The figure shows three views and two pictorial views of one solid part (mm, origin at its lowest corner). Answer the questions. Give positions to 0.01 mm unless a question says otherwise; leave off trailing zeros. Loops run counter-clockwise (first coordinate to the right, second up) from the corner with the lowest first, then second, coordinate; pieces in that order, holes last. Notation, with made-up numbers: (34.5, 54.25) - (41.5, 54.25) arc R21 ccw to (41.5, 78.25) - close; hole circle Ø11 at (-3.75, 59). An arc over 180 degrees is marked (long way). Use CSV: the item, a comma, the result in double quotes.
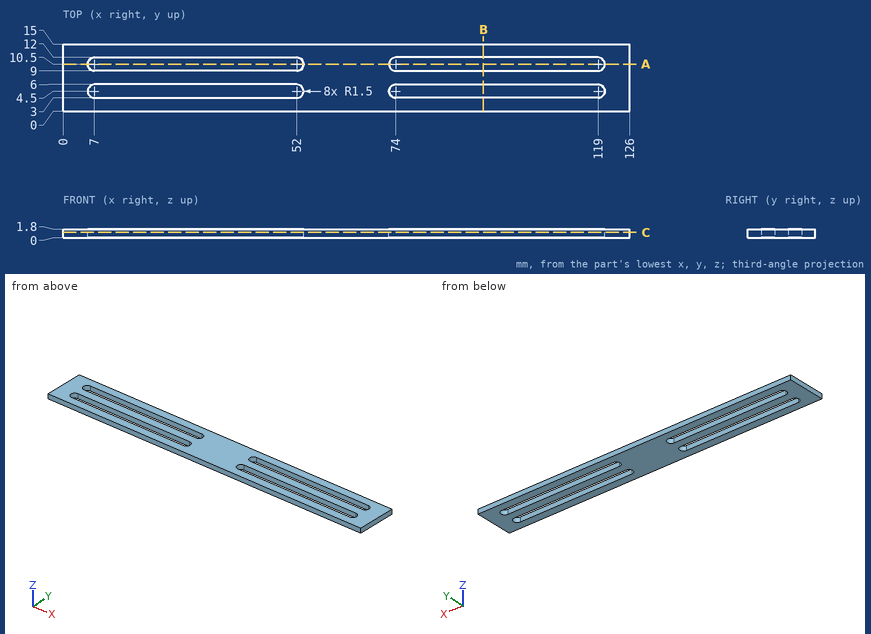
Item 1: A cutting plane is placed at C-C on z = 1.15. Determine the outline of the cut face in (x, y).
Determined:
outline,"(0, 0) - (126, 0) - (126, 15) - (0, 15) - close; hole (7, 3) - (52, 3) arc R1.5 ccw to (52, 6) - (7, 6) arc R1.5 ccw to start; hole (7, 9) - (52, 9) arc R1.5 ccw to (52, 12) - (7, 12) arc R1.5 ccw to start; hole (74, 3) - (119, 3) arc R1.5 ccw to (119, 6) - (74, 6) arc R1.5 ccw to start; hole (74, 9) - (119, 9) arc R1.5 ccw to (119, 12) - (74, 12) arc R1.5 ccw to start"
Item 2: A cutting plane is placed at A-A on y = 10.5. Determine the outline of the cut face in (x, z), and give its area (3 significant figures).
Determined:
outline,"(0, 0) - (5.5, 0) - (5.5, 1.8) - (0, 1.8) - close; (53.5, 0) - (72.5, 0) - (72.5, 1.8) - (53.5, 1.8) - close; (120.5, 0) - (126, 0) - (126, 1.8) - (120.5, 1.8) - close"
area,"54.0 mm²"
Item 3: A cutting plane is placed at B-B on x = 93.5. Determine the outline of the cut face in (y, z), and give its area (3 significant figures).
Determined:
outline,"(0, 0) - (3, 0) - (3, 1.8) - (0, 1.8) - close; (6, 0) - (9, 0) - (9, 1.8) - (6, 1.8) - close; (12, 0) - (15, 0) - (15, 1.8) - (12, 1.8) - close"
area,"16.2 mm²"
Item 4: Find the intervals of material crossed by line 1 (Y direction, x = 46, z = 1); line 2 (X direction, y = 5, z = 1.55), in increasing order.
Determined:
line 1,"y = 0 to 3, 6 to 9, 12 to 15"
line 2,"x = 0 to 5.59, 53.41 to 72.59, 120.41 to 126"
